Design review of the part built by this model. Coordinates are the model's own, in mm. A direction names the side the tool comes from. Coordinates: 2 decimals unless noted, no trailing zeros. Loops run counter-clockwise (first coordinate to the right, second up) from the corner with the lowest first, then second, coordinate; pieces in that order, holes last. Notation, with made-up numbers: M 35,-33.5 L 63,-33.5 A20 cw 63,-2.5 Z; hole C -1,-27.5 d5. An arc over 180 degrees is marked long. One line per item, written item: value.
```python
from build123d import *

# Parameters (mm, degrees)
SKETCH1_R               = 155
BOSS_EXTRUDE1_DEPTH     = 75
SKETCH2_R               = 142.5
CUT_EXTRUDE1_DEPTH      = 25
SKETCH3_R               = 85
BOSS_EXTRUDE2_DEPTH     = 37
SKETCH4_R               = 80
BOSS_EXTRUDE3_DEPTH     = 105
CUT_EXTRUDE2_DEPTH      = 292.400068634
CUT_EXTRUDE2_DEPTH_BACK = 292.400068634
SKETCH6_R               = 75
BOSS_EXTRUDE4_DEPTH     = 5
SKETCH7_R               = 60
CUT_EXTRUDE3_DEPTH      = 58
SKETCH8_R               = 12.5
CUT_EXTRUDE4_DEPTH      = 262.178100154


with BuildPart() as part:
    # Sketch1 → Boss-Extrude1 (new body)
    with BuildSketch(Plane(origin=(0, 0, 0), x_dir=(1, 0, 0), z_dir=(0, 1, 0))):
        with Locations(Location((0, 0, 0), (0, 0, 270))):
            Circle(SKETCH1_R)
    extrude(amount=BOSS_EXTRUDE1_DEPTH)

    # Sketch2 → Cut-Extrude1 (cut)
    with BuildSketch(Plane(origin=(0, 75, 0), x_dir=(1, 0, 0), z_dir=(0, 1, 0))):
        with Locations(Location((0, 0, 0), (0, 0, 270))):
            Circle(SKETCH2_R)
    extrude(amount=-CUT_EXTRUDE1_DEPTH, mode=Mode.SUBTRACT)

    # Sketch3 → Boss-Extrude2 (add)
    with BuildSketch(Plane(origin=(0, 50, 0), x_dir=(1, 0, 0), z_dir=(0, 1, 0))):
        with Locations(Location((0, 0, 0), (0, 0, 270))):
            Circle(SKETCH3_R)
    extrude(amount=BOSS_EXTRUDE2_DEPTH)

    # Sketch4 → Boss-Extrude3 (add)
    with BuildSketch(Plane(origin=(0, 87, 0), x_dir=(1, 0, 0), z_dir=(0, 1, 0))):
        with Locations(Location((0, 0, 0), (0, 0, 270))):
            Circle(SKETCH4_R)
    extrude(amount=BOSS_EXTRUDE3_DEPTH)

    # Sketch5 → Cut-Extrude2 (cut, two sides: drawn at the far end of the back side and taken through both)
    with BuildSketch(Plane(origin=(0, 192, 0), x_dir=(1, 0, 0), z_dir=(0, 1, 0)).offset(-CUT_EXTRUDE2_DEPTH_BACK)):
        with BuildLine():
            Line((33.541019662, 10), (41.541019662, 10))
            Line((41.541019662, 10), (41.541019662, -10))
            Line((41.541019662, -10), (33.541019662, -10))
            ThreePointArc((33.541019662, -10), (-35, 0), (33.541019662, 10))
        make_face()
    extrude(amount=CUT_EXTRUDE2_DEPTH + CUT_EXTRUDE2_DEPTH_BACK, mode=Mode.SUBTRACT)

    # Sketch6 → Boss-Extrude4 (add)
    with BuildSketch(Plane.XZ):
        with Locations(Location((0, 0, 0), (0, 0, 90))):
            Circle(SKETCH6_R)
    extrude(amount=BOSS_EXTRUDE4_DEPTH)

    # Sketch7 → Cut-Extrude3 (cut)
    with BuildSketch(Plane.XZ.offset(5)):
        with Locations(Location((0, 0, 0), (0, 0, 270))):
            Circle(SKETCH7_R)
    extrude(amount=-CUT_EXTRUDE3_DEPTH, mode=Mode.SUBTRACT)

    # Sketch8 → Cut-Extrude4 (cut, through all)
    with BuildSketch(Plane(origin=(0, 50, 0), x_dir=(1, 0, 0), z_dir=(0, 1, 0))):
        with Locations(Location((0, 115.062551677, 0), (0, 0, 270))):
            Circle(SKETCH8_R)
        with Locations(Location((99.647092776, 57.531275838, 0), (0, 0, 270))):
            Circle(SKETCH8_R)
        with Locations(Location((99.647092776, -57.531275838, 0), (0, 0, 270))):
            Circle(SKETCH8_R)
        with Locations(Location((0, -115.062551677, 0), (0, 0, 270))):
            Circle(SKETCH8_R)
        with Locations(Location((-99.647092776, -57.531275838, 0), (0, 0, 270))):
            Circle(SKETCH8_R)
        with Locations(Location((-99.647092776, 57.531275838, 0), (0, 0, 270))):
            Circle(SKETCH8_R)
    extrude(amount=-CUT_EXTRUDE4_DEPTH, mode=Mode.SUBTRACT)


solid = part.part
```
(1) To check wall thickness, follow line 1 along X through (y, z) = (124.5, 0); line 2 along X through (y, z) = (64.25, 0); line 3 along Y through (x, z) = (-81.5, -33). State the ranges of each line that lie inside material, in increasing order. Write a range as [from, to].
Reply:
line 1: x = [-80, -35], [41.54, 80]
line 2: x = [-155, -142.5], [-85, -35], [41.54, 85], [142.5, 155]
line 3: y = [0, 50]
(2) We need section C-C on y = 112. State the section outline as (x, z) points, then the cut area to 3 significant figures.
Reply:
outline: C 0,0 d160; hole M 33.54,-10 L 41.54,-10 L 41.54,10 L 33.54,10 A35 ccw long Z
area: 16,100 mm2
(3) Mouldability with a two-part tool opening along Z and no side actions: class faces 1 (the flat face through (41.541, 122, 0)), 2 (the flat face through (-67, 0, -37)), 3 (the cylindrical face through (-59.37, 36.98, 143.18)) as released by +Z, released by -Z, zero draft, split by the parting line, or undercut.
Reply:
face 1: undercut
face 2: zero draft
face 3: split by the parting line
(4) Tool access review of faces 4 (the flat face through (-34, 192, 17)), 5 (the cylindrical face through (45.636, -2.465, -59.517)), 6 (the flat face through (38, 122, 10)), 7 (the flat face through (-126, 75, 68)), 8 (the flat face through (-50, -5, -34)): name each direction out of +Z, -Z, +X, -X, +Y, -Y from which nothing blocks a thin tool from reaching the whole face with its end or side.
Reply:
face 4: +Z, -Z, +X, -X, +Y
face 5: -Y
face 6: +Y, -Y
face 7: +Y
face 8: +Z, -Z, +X, -X, -Y
(5) Insertion check: pin 1 (6.5 mm diameter, centred on x = 36, y = 156.5, fed in from +Z); pin 2 (6 mm diameter, centred on x = 76, z = -60, fed in from -Y); pin 3 (10 mm diameter, centred on y = 94.5, z = 11.5, fed in from +X). Each pin has a flat end and moves straight along its axis. Give the tip position at first contact, or say it passes through.
Reply:
pin 1: stops at z = 72.99
pin 2: stops at y = 0
pin 3: stops at x = 79.74
(6) We need section A-A on z = 0. State the section outline as (x, y) points.
Reply:
outline: M -155,0 L -75,0 L -75,-5 L -60,-5 L -60,53 L -35,53 L -35,192 L -80,192 L -80,87 L -85,87 L -85,50 L -142.5,50 L -142.5,75 L -155,75 Z; M 41.54,53 L 60,53 L 60,-5 L 75,-5 L 75,0 L 155,0 L 155,75 L 142.5,75 L 142.5,50 L 85,50 L 85,87 L 80,87 L 80,192 L 41.54,192 Z
(7) We need section D-D on x = 0. State how many separate pieces and enclosed holes the cut face has, then the cut area to 3 significant figures.
Reply:
separate pieces: 4
enclosed holes: 0
area: 20,800 mm2
(8) We need section B-B on x = -95.5. State the section outline as (y, z) points, then the cut area to 3 significant figures.
Reply:
outline: M 0,-122.09 L 75,-122.09 L 75,-105.76 L 50,-105.76 L 50,-69.32 L 0,-69.32 Z; M 0,-45.74 L 50,-45.74 L 50,45.74 L 0,45.74 Z; M 0,69.32 L 50,69.32 L 50,105.76 L 75,105.76 L 75,122.09 L 0,122.09 Z
area: 10,700 mm2
